Part model, mm, in its own coordinate system. Give positions to 0.01 mm unless a question says otherwise; leave off trailing zeros. Order: outer loops, then holes, each group sorted by start corner. A loop starts at its lowest first (then second) coordinate and runs counter-clockwise, first axis right, second up. Notation, with made-up numbers: M 3,-13.5 L 27,-13.5 A15 ccw 27,4.5 Z; hole C 63,0 d9. An arc over 180 degrees is marked long. Return JSON: item names as keys, results as strings.
from build123d import *

# Parameters (mm, degrees)
BOSS_EXTRUDE1_DEPTH = 30
SKETCH2_R           = 1.853585504
SKETCH2_R_2         = 2.5
CUT_EXTRUDE1_DEPTH  = 18


with BuildPart() as part:
    # Sketch1 → Boss-Extrude1 (new body)
    with BuildSketch(Plane(origin=(0, 0, 0), x_dir=(1, 0, 0), z_dir=(0, 1, 0))):
        with BuildLine():
            Line((-79.094879733, 12), (-75, 12))
            Line((-75, 12), (-75, -12))
            Line((-75, -12), (-79.094879733, -12))
            ThreePointArc((-79.094879733, -12), (-80, 0), (-79.094879733, 12))
        make_face()
    extrude(amount=BOSS_EXTRUDE1_DEPTH)

    # Sketch2 → Cut-Extrude1 (cut)
    with BuildSketch(Plane(origin=(-75, 0, 0), x_dir=(0, 0, -1), z_dir=(1, 0, 0))):
        with Locations((0, 15)):
            Circle(SKETCH2_R)
        with Locations((6.187184335, 21.187184335)):
            Circle(SKETCH2_R_2)
        with Locations((6.187184335, 8.812815665)):
            Circle(SKETCH2_R_2)
        with Locations((-6.187184335, 8.812815665)):
            Circle(SKETCH2_R_2)
        with Locations((-6.187184335, 21.187184335)):
            Circle(SKETCH2_R_2)
    extrude(amount=-CUT_EXTRUDE1_DEPTH, mode=Mode.SUBTRACT)


solid = part.part
Q1. Pin check, flat tips, straight feed: pin 1 (6.5 mm diameter, centred on y = 8.81, z = 6.19, fed in from +X); pin 2 (6 mm diameter, centred on y = 8.81, z = -6.19, fed in from -X); pin 3 (8 mm diameter, centred on y = 27, z = -9, fed in from -X). Stop position of each tip, or through.
Established:
{"pin 1": "stops at x = -75", "pin 2": "stops at x = -79.94", "pin 3": "stops at x = -79.84"}
Q2. Two-plate mould, pull along Y, no slides. Class faces 1 (the cylindrical face through (-77.423, 21.938, 3.803)), 2 (the cylindrical face through (-77.423, 7.855, 3.878)), 3 (the flat face through (-77, 0, 0)), 4 (the flat face through (-75, 14.8, 2.5)): +Y half, -Y half, draft (parallel to the pull), parting line (faces both ways), or undercut.
Established:
{"face 1": "undercut", "face 2": "undercut", "face 3": "-Y half", "face 4": "draft"}
Q3. Band-saw the part on D-D (y = 21.5). Give the cut face in (x, z), then the cut area to 3 significant figures.
Established:
{"outline": "M -79.91,-3.71 L -75,-3.71 L -75,3.71 L -79.91,3.71 A80 ccw Z; M -79.53,-8.67 A80 ccw -79.09,-12 L -75,-12 L -75,-8.67 Z; M -79.53,8.67 L -75,8.67 L -75,12 L -79.09,12 A80 ccw Z", "area": "65.7 mm²"}
Q4. Band-saw the part on A-A (z = 0). Give the cut face in (x, y), then the cut area to 3 significant figures.
Established:
{"outline": "M -80,0 L -75,0 L -75,13.15 L -80,13.15 Z; M -80,16.85 L -75,16.85 L -75,30 L -80,30 Z", "area": "131 mm²"}
Q5. Band-saw the part on B-B (y = 16.5). Give the cut face in (x, z), then the cut area to 3 significant figures.
Established:
{"outline": "M -79.99,-1.09 A80 ccw -79.09,-12 L -75,-12 L -75,-1.09 Z; M -79.99,1.09 L -75,1.09 L -75,12 L -79.09,12 A80 ccw Z", "area": "102 mm²"}
Q6. Probe line 1 along Z through (x, y) = (-77.05, 9); line 2 along Z through (x, y) = (-75.9, 19); line 3 along Y through (x, z) = (-78.45, 0). List the from-to ranges inside material, lowest first.
Established:
{"line 1": "z = -12 to -8.68, -3.69 to 3.69, 8.68 to 12", "line 2": "z = -12 to -7.4, -4.98 to 4.98, 7.4 to 12", "line 3": "y = 0 to 13.15, 16.85 to 30"}
Q7. Band-saw the part on C-C (z = 5.25). Give the cut face in (x, y), then the cut area to 3 significant figures.
Established:
{"outline": "M -79.83,0 L -75,0 L -75,6.5 L -79.83,6.5 Z; M -79.83,11.13 L -75,11.13 L -75,18.87 L -79.83,18.87 Z; M -79.83,23.5 L -75,23.5 L -75,30 L -79.83,30 Z", "area": "100 mm²"}
